```python
from build123d import *

# Parameters (mm, degrees)
SKETCH1_R           = 15.9
SKETCH1_R_2         = 5
SKETCH1_R_3         = 1.625
BOSS_EXTRUDE1_DEPTH = 3.88
SKETCH2_R           = 8
SKETCH2_R_2         = 5
BOSS_EXTRUDE2_DEPTH = 15
CHAMFER1_SIZE       = 0.5


with BuildPart() as part:
    # Sketch1 → Boss-Extrude1 (new body)
    with BuildSketch(Plane.XY):
        Circle(SKETCH1_R)
        Circle(SKETCH1_R_2, mode=Mode.SUBTRACT)
        with Locations((0, 12.025)):
            Circle(SKETCH1_R_3, mode=Mode.SUBTRACT)
        with Locations((12.025, 0)):
            Circle(SKETCH1_R_3, mode=Mode.SUBTRACT)
        with Locations((0, -12.025)):
            Circle(SKETCH1_R_3, mode=Mode.SUBTRACT)
        with Locations((-12.025, 0)):
            Circle(SKETCH1_R_3, mode=Mode.SUBTRACT)
    extrude(amount=BOSS_EXTRUDE1_DEPTH)

    # Sketch2 → Boss-Extrude2 (add)
    with BuildSketch(Plane.XY.offset(3.88)):
        Circle(SKETCH2_R)
        Circle(SKETCH2_R_2, mode=Mode.SUBTRACT)
    extrude(amount=BOSS_EXTRUDE2_DEPTH)

    # Chamfer1
    chamfer1_edges = [part.edges().sort_by_distance(p)[0] for p in [
        (-15.9, 0, 0),
        (-8, 0, 18.88),
        (-8, 0, 3.88),
        (-5, 0, 18.88),
        (-15.9, 0, 3.88),
    ]]
    chamfer(chamfer1_edges, length=CHAMFER1_SIZE)


solid = part.part
```
Input: part model. Units: mm. Frame: model coordinates. A direction names the side the tool comes from. Coordinates: 2 decimals unless noted, no trailing zeros. Loops run counter-clockwise (first coordinate to the right, second up) from the corner with the lowest first, then second, coordinate; pieces in that order, holes last. Notation, with made-up numbers: M 22,19 L 52,19 A33 ccw 52,47 Z; hole C 28,82 d1. An arc over 180 degrees is marked long. Answer in a Markdown table with one row per item.
1. Draft query along Y for faces 1 (the cylindrical face through (-0.212, -10.414, 1.913)), 2 (the flat face through (-4, 4, 18.88)), 3 (the cylindrical face through (-3.45, -15.52, 1.92)). Return one class per face: pulls with the +Y half, pulls with the -Y half, needs draft (parallel to the pull), parting line crosses it, or undercut.
Response:
| item | result |
|---|---|
| face 1 | undercut |
| face 2 | needs draft |
| face 3 | parting line crosses it |
2. First-contact query: pin 1 (5 mm diameter, centred on x = 0, y = 12.025, fed in from +Z); pin 2 (2 mm diameter, centred on x = 4.5, z = 11, fed in from +Y); pin 3 (10 mm diameter, centred on y = 5, z = 15.5, fed in from +X). Flat tips, straight axial feed; report the tip coordinate or a pass-through.
Response:
| item | result |
|---|---|
| pin 1 | stops at z = 3.88 |
| pin 2 | stops at y = 7.19 |
| pin 3 | stops at x = 8 |
3. Section A-A, the plane x = 0. Count the separate pieces of the cut face and the enclosed holes in it, then the cut area to 3 significant figures.
Response:
| item | result |
|---|---|
| separate pieces | 4 |
| enclosed holes | 0 |
| area | 149 mm2 |
4. Reachability of faces 4 (the cylindrical face through (-1.73, -7.81, 11.28)), 5 (the cylindrical face through (-13.65, 0.07, 1.91)) from +Z, -Z, +X, -X, +Y, -Y: full face, straight path, thin tool, end or side. Return the list, or none.
Response:
| item | result |
|---|---|
| face 4 | +Z |
| face 5 | +Z, -Z |
5. Section B-B, the plane z = 16.75. Output: boundary loops of the cut face in (x, y), then the cut area to 3 significant figures.
Response:
| item | result |
|---|---|
| outline | C 0,0 d16; hole C 0,0 d10 |
| area | 123 mm2 |
6. Section D-D, the plane z = 2. Output: boundary loops of the cut face in (x, y) (3 decimals), then the cut area to 3 significant figures.
Response:
| item | result |
|---|---|
| outline | C 0,0 d31.8; hole C -12.025,0 d3.25; hole C 0,0 d10; hole C 0,-12.025 d3.25; hole C 0,12.025 d3.25; hole C 12.025,0 d3.25 |
| area | 683 mm2 |
7. Material intervals for line 1 (Y direction, x = 0, z = 2.75); line 2 (Z direction, x = -7.5, y = -13); line 3 (X direction, y = 2, z = 7.5), sorted ascending.
Response:
| item | result |
|---|---|
| line 1 | y = -15.9 to -13.65, -10.4 to -5, 5 to 10.4, 13.65 to 15.9 |
| line 2 | z = 0 to 3.88 |
| line 3 | x = -7.75 to -4.58, 4.58 to 7.75 |
